The listing builds one solid part. Answer for the finished solid, in the listing's coordinates (mm). Face numbers are marked on the shaded views. Give positions to 0.01 mm unless a question says otherwise; leave off trailing zeros. Order: outer loops, then holes, each group sorted by start corner. A loop starts at its lowest first (then second) coordinate and runs counter-clockwise, first axis right, second up. Notation, with made-up numbers: M -29,-35.75 L 10,-35.75 A19 ccw 10,-18.75 Z; hole C 55,19.5 d5. An arc over 180 degrees is marked long. Answer as a JSON object with one key per item and string values. Group by question number.
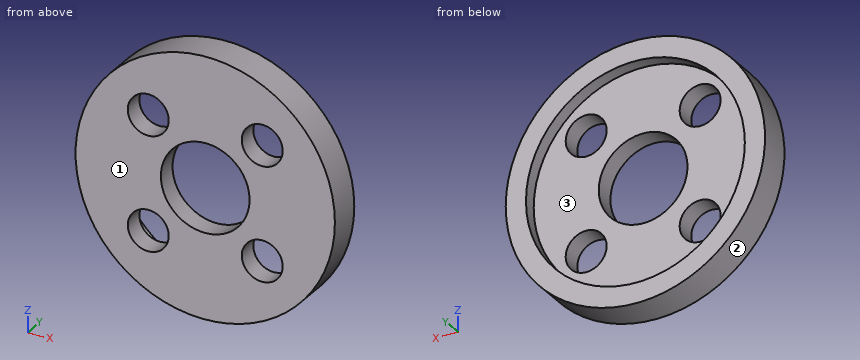
```python
from build123d import *

# Parameters (mm, degrees)
SKETCH1_R           = 105
BOSS_EXTRUDE1_DEPTH = 40
SKETCH3_R           = 6.5
CUT_EXTRUDE2_DEPTH  = 40
SKETCH4_R           = 16.035
CUT_EXTRUDE3_DEPTH  = 5
SKETCH8_R           = 3
CUT_EXTRUDE6_DEPTH  = 44.5
SKETCH11_R          = 90
SKETCH11_R_2        = 26.035
CUT_EXTRUDE8_DEPTH  = 10
SKETCH12_R          = 108
SKETCH12_R_2        = 105
BOSS_EXTRUDE2_DEPTH = 3
SKETCH13_R          = 108
SKETCH13_R_2        = 19
CUT_EXTRUDE9_DEPTH  = 41
SKETCH14_R          = 27.444507403
CUT_EXTRUDE10_DEPTH = 32
SKETCH15_R          = 19
CUT_EXTRUDE11_DEPTH = 3


with BuildPart() as part:
    # Sketch1 → Boss-Extrude1 (new body)
    with BuildSketch(Plane(origin=(0, 0, 0), x_dir=(1, 0, 0), z_dir=(0, 1, 0))):
        Circle(SKETCH1_R)
    extrude(amount=BOSS_EXTRUDE1_DEPTH)

    # Sketch3 → Cut-Extrude2 (cut)
    with BuildSketch(Plane(origin=(0, 40, 0), x_dir=(1, 0, 0), z_dir=(0, 1, 0))):
        Circle(SKETCH3_R)
    extrude(amount=-CUT_EXTRUDE2_DEPTH, mode=Mode.SUBTRACT)

    # Sketch4 → Cut-Extrude3 (cut)
    with BuildSketch(Plane(origin=(0, 40, 0), x_dir=(1, 0, 0), z_dir=(0, 1, 0))):
        Circle(SKETCH4_R)
    extrude(amount=-CUT_EXTRUDE3_DEPTH, mode=Mode.SUBTRACT)

    # Sketch8 → Cut-Extrude6 (cut)
    with BuildSketch(Plane(origin=(0, 35, 0), x_dir=(1, 0, 0), z_dir=(0, 1, 0))):
        with Locations((-8.35, 8.35)):
            Circle(SKETCH8_R)
        with Locations((8.35, 8.35)):
            Circle(SKETCH8_R)
        with Locations((8.35, -8.35)):
            Circle(SKETCH8_R)
        with Locations((-8.35, -8.35)):
            Circle(SKETCH8_R)
    extrude(amount=-CUT_EXTRUDE6_DEPTH, mode=Mode.SUBTRACT)

    # Sketch11 → Cut-Extrude8 (cut)
    with BuildSketch(Plane(origin=(0, 40, 0), x_dir=(1, 0, 0), z_dir=(0, 1, 0))):
        Circle(SKETCH11_R)
        Circle(SKETCH11_R_2, mode=Mode.SUBTRACT)
    extrude(amount=-CUT_EXTRUDE8_DEPTH, mode=Mode.SUBTRACT)

    # Sketch12 → Boss-Extrude2 (add)
    with BuildSketch(Plane(origin=(0, 40, 0), x_dir=(1, 0, 0), z_dir=(0, 1, 0))):
        Circle(SKETCH12_R)
        Circle(SKETCH12_R_2, mode=Mode.SUBTRACT)
    boss_extrude2 = extrude(amount=-BOSS_EXTRUDE2_DEPTH)

    # Mirror1: Boss-Extrude2 across plane
    add(boss_extrude2.mirror(Plane(origin=(0, 20, 0), x_dir=(0, 0, 1), z_dir=(0, -1, 0))))

    # Sketch13 → Cut-Extrude9 (cut, through all)
    with BuildSketch(Plane(origin=(0, 40, 0), x_dir=(1, 0, 0), z_dir=(0, 1, 0))):
        Circle(SKETCH13_R)
        Circle(SKETCH13_R_2, mode=Mode.SUBTRACT)
    extrude(amount=-CUT_EXTRUDE9_DEPTH, mode=Mode.SUBTRACT)

    # Sketch14 → Cut-Extrude10 (cut)
    with BuildSketch(Plane.XZ):
        Circle(SKETCH14_R)
    extrude(amount=-CUT_EXTRUDE10_DEPTH, mode=Mode.SUBTRACT)

    # Sketch15 → Cut-Extrude11 (cut)
    with BuildSketch(Plane(origin=(0, 40, 0), x_dir=(1, 0, 0), z_dir=(0, 1, 0))):
        Circle(SKETCH15_R)
    extrude(amount=-CUT_EXTRUDE11_DEPTH, mode=Mode.SUBTRACT)


solid = part.part
```
Item 1: Section C-C (y = 33.05) is taken. Determine the outline of the cut face in (x, z).
Item 2: Section B-B (z = 3.5) is taken. Determine the outline of the cut face in (x, y).
Item 3: Section D-D (x = 0) is taken. Determine the outline of the cut face in (y, z) (3 decimals), and give its area (3 significant figures).
Item 4: Section A-A (x = -8.35) is taken. Determine the outline of the cut face in (y, z).
Item 5: Determine the mould class of the marked faces 1, 2 and 3 for opening direction X: released by +X, released by -X, zero draft, split by the parting line, or undercut.
Item 6: Consider probe 1 along Z at (x, y) = (0, 35.8) (3 decimals); probe 2 along X at (y, z) = (32.65, -8.35); probe 3 along X at (y, z) = (32.9, 0). Determine where each line is inside the solid, lowest interval first. Write a range as from..to.
Item 7: Flat-ended cylindrical pins translate along their axes: P1, Ø1.5, axis at x = 12.5, y = 36, coming from the -Z side; P2, Ø8, axis at x = -8.35, z = -8.35, coming from the +Y side; P3, Ø1.5, axis at x = -10.5, y = 35.5, coming from the +Z side. Find the tip coordinate at first contact, or state that the pin passes through.
Values found:
{
 "1": {"outline": "C 0,0 d38; hole C -8.35,-8.35 d6; hole C -8.35,8.35 d6; hole C 0,0 d13; hole C 8.35,-8.35 d6; hole C 8.35,8.35 d6"},
 "2": {"outline": "M -18.67,32 L -5.48,32 L -5.48,35 L -15.65,35 L -15.65,37 L -18.67,37 Z; M 5.48,32 L 18.67,32 L 18.67,37 L 15.65,37 L 15.65,35 L 5.48,35 Z"},
 "3": {"outline": "M 32,-19 L 37,-19 L 37,-16.035 L 35,-16.035 L 35,-6.5 L 32,-6.5 Z; M 32,6.5 L 35,6.5 L 35,16.035 L 37,16.035 L 37,19 L 32,19 Z", "area": "86.9 mm^2"},
 "4": {"outline": "M 32,-17.07 L 37,-17.07 L 37,-13.69 L 35,-13.69 L 35,-11.35 L 32,-11.35 Z; M 32,-5.35 L 35,-5.35 L 35,5.35 L 32,5.35 Z; M 32,11.35 L 35,11.35 L 35,13.69 L 37,13.69 L 37,17.07 L 32,17.07 Z"},
 "5": {"face 1": "zero draft", "face 2": "split by the parting line", "face 3": "undercut"},
 "6": {"probe 1": "z = -19..-16.035, 16.035..19", "probe 2": "x = -17.07..-11.35, -5.35..5.35, 11.35..17.07", "probe 3": "x = -19..-6.5, 6.5..19"},
 "7": {"P1": "stops at z = -14.93", "P2": "stops at y = 35", "P3": "stops at z = 16.31"}
}
